The model under review builds one solid part; all positions refer to its coordinate system, in mm. A direction names the side the tool comes from. Coordinates: 2 decimals unless noted, no trailing zeros. Loops run counter-clockwise (first coordinate to the right, second up) from the corner with the lowest first, then second, coordinate; pieces in that order, holes last. Notation, with made-up numbers: M 87,61.25 L 103,61.25 A24 cw 103,98.25 Z; hole C 29,41 d3. An arc over 180 degrees is marked long. Use CSV: the item, a comma, the result in double quotes. Start each with the question number.
1. Draft analysis for pull direction X (two halves, no side actions). For faces 1 (the cylindrical face through (26, 12, 3)), 2 (the flat face through (-17.4, 5.5, 5.7)), 3 (the cylindrical face through (-26, 12, 3)), 4 (the flat face through (17.4, -8.5, 5.7)), state which applies: +X half, -X half, draft (parallel to the pull), parting line (faces both ways), or undercut.
2. Tool access review of faces 5 (the flat face through (22.6, 8.5, 5.7)), 6 (the flat face through (26.37, 0.13, 6.88)): name each direction out of +Z, -Z, +X, -X, +Y, -Y from which nothing blocks a thin tool from reaching the whole face with its end or side.
3. Add section C-C, the plane z = 5.5. State how many separate pieces and enclosed holes the cut face has, then the cut area to 3 significant figures.
4. For L1, parallel to Y at x = -20, z = 0.95; L2, parallel to Y at x = -21, z = 4.25; L3, parallel to X at y = -6.5, z = 4.5, list the stretches that pass through material, from the lowest coordinate up.
5. Clearance check with a flat-ended pin moving along its axis: P1, Ø1.8, axis at x = -21.5, y = -5.5, coming from the +Z side. State where the tip first meets the part, or that it passes through.
6. Add section A-A, the plane z = 2.75. Write out the cut boundary in (x, y).
7. Add section B-B, the plane x = 20. Write out the cut boundary in (y, z).
from build123d import *

# Parameters (mm, degrees)
BASE_W              = 54
BASE_H              = 28
BASE_R              = 1.55
BOSS_EXTRUDE1_DEPTH = 4
BOSS_EXTRUDE2_START = 4
BASE_3_W            = 54
BASE_3_H            = 28
BOSS_EXTRUDE2_DEPTH = 3.5
FILLET1_R           = 5
CHAMFER1_SIZE       = 1.25


with BuildPart() as part:
    # Base → Boss-Extrude1 (new body)
    with BuildSketch(Plane.XY):
        Rectangle(BASE_W, BASE_H)
        with Locations((-20, 7)):
            Circle(BASE_R, mode=Mode.SUBTRACT)
        with Locations((20, 7)):
            Circle(BASE_R, mode=Mode.SUBTRACT)
        with Locations((20, -7)):
            Circle(BASE_R, mode=Mode.SUBTRACT)
        with Locations((-20, -7)):
            Circle(BASE_R, mode=Mode.SUBTRACT)
    extrude(amount=BOSS_EXTRUDE1_DEPTH)

    # Base<3> → Boss-Extrude2 (add)
    with BuildSketch(Plane.XY.offset(BOSS_EXTRUDE2_START)):
        Rectangle(BASE_3_W, BASE_3_H)
        Polygon((-21.732050808, -10), (-18.267949192, -10), (-16.535898385, -7), (-18.267949192, -4), (-21.732050808, -4), (-23.464101615, -7), align=None, mode=Mode.SUBTRACT)
        Polygon((21.732050808, -10), (23.464101615, -7), (21.732050808, -4), (18.267949192, -4), (16.535898385, -7), (18.267949192, -10), align=None, mode=Mode.SUBTRACT)
        Polygon((21.732050808, 4), (23.464101615, 7), (21.732050808, 10), (18.267949192, 10), (16.535898385, 7), (18.267949192, 4), align=None, mode=Mode.SUBTRACT)
        Polygon((-18.267949192, 4), (-16.535898385, 7), (-18.267949192, 10), (-21.732050808, 10), (-23.464101615, 7), (-21.732050808, 4), align=None, mode=Mode.SUBTRACT)
    extrude(amount=BOSS_EXTRUDE2_DEPTH)

    # Fillet1
    fillet1_edges = [part.edges().sort_by_distance(p)[0] for p in [
        (27, 14, 3.75),
        (27, -14, 3.75),
        (-27, -14, 3.75),
        (-27, 14, 3.75),
    ]]
    fillet(fillet1_edges, radius=FILLET1_R)

    # Chamfer1
    chamfer1_edges = [part.edges().sort_by_distance(p)[0] for p in [
        (-27, 0, 7.5),
        (0, 14, 7.5),
        (0, -14, 7.5),
        (27, 0, 7.5),
        (-25.535533906, -12.535533906, 7.5),
        (25.535533906, -12.535533906, 7.5),
        (25.535533906, 12.535533906, 7.5),
        (-25.535533906, 12.535533906, 7.5),
    ]]
    chamfer(chamfer1_edges, length=CHAMFER1_SIZE)


solid = part.part
Computed:
1,face 1,"+X half"
1,face 2,"undercut"
1,face 3,"-X half"
1,face 4,"undercut"
2,face 5,"+Z"
2,face 6,"+Z, +X, +Y, -Y"
3,separate pieces,"1"
3,enclosed holes,"4"
3,area,"1,370 mm^2"
4,L1,"y = -14 to -8.55, -5.45 to 5.45, 8.55 to 14"
4,L2,"y = -14 to -10, -4 to 4, 10 to 14"
4,L3,"x = -27 to -23.18, -16.82 to 16.82, 23.18 to 27"
5,P1,"stops at z = 4"
6,outline,"M -27,-9 A5 ccw -22,-14 L 22,-14 A5 ccw 27,-9 L 27,9 A5 ccw 22,14 L -22,14 A5 ccw -27,9 Z; hole C -20,-7 d3.1; hole C -20,7 d3.1; hole C 20,-7 d3.1; hole C 20,7 d3.1"
7,outline,"M -14,0 L -8.55,0 L -8.55,4 L -10,4 L -10,7.5 L -12.75,7.5 L -14,6.25 Z; M -5.45,0 L 5.45,0 L 5.45,4 L 4,4 L 4,7.5 L -4,7.5 L -4,4 L -5.45,4 Z; M 8.55,0 L 14,0 L 14,6.25 L 12.75,7.5 L 10,7.5 L 10,4 L 8.55,4 Z"
